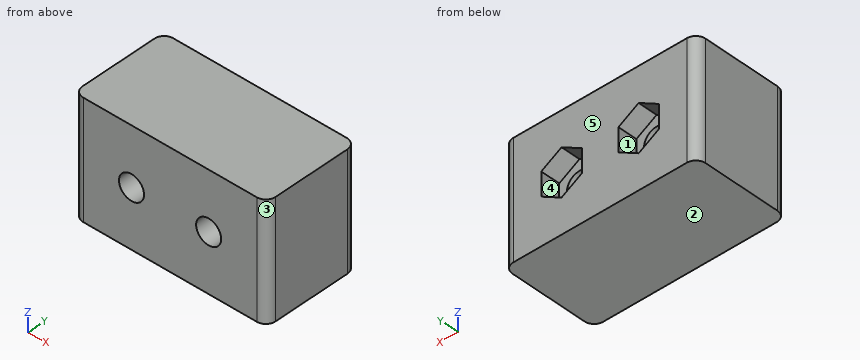
```python
from build123d import *

# Parameters (mm, degrees)
BOSS_EXTRUDE1_DEPTH = 6
SKETCH2_R           = 1.3
CUT_EXTRUDE1_DEPTH  = 10
CUT_EXTRUDE2_DEPTH  = 2


with BuildPart() as part:
    # Sketch1 → Boss-Extrude1 (new, symmetric)
    with BuildSketch(Plane.XY):
        with BuildLine():
            Line((-9, 0), (9, 0))
            ThreePointArc((9, 0), (9.707106781, 0.292893219), (10, 1))
            Line((10, 1), (10, 9))
            ThreePointArc((10, 9), (9.707106781, 9.707106781), (9, 10))
            Line((9, 10), (-9, 10))
            ThreePointArc((-9, 10), (-9.707106781, 9.707106781), (-10, 9))
            Line((-10, 9), (-10, 1))
            ThreePointArc((-10, 1), (-9.707106781, 0.292893219), (-9, 0))
        make_face()
    extrude(amount=BOSS_EXTRUDE1_DEPTH, both=True)

    # Sketch2 → Cut-Extrude1 (cut)
    with BuildSketch(Plane(origin=(0, 0, 0), x_dir=(1, 0, 0), z_dir=(0, 1, 0))):
        with Locations(Location((4, 0, 0), (0, 0, 270))):
            Circle(SKETCH2_R)
        with Locations(Location((-4, 0, 0), (0, 0, 270))):
            Circle(SKETCH2_R)
    extrude(amount=CUT_EXTRUDE1_DEPTH, mode=Mode.SUBTRACT)

    # Sketch3 → Cut-Extrude2 (cut)
    with BuildSketch(Plane(origin=(0, 10, 0), x_dir=(1, 0, 0), z_dir=(0, 1, 0))):
        Polygon((6.1, -1.212435565), (4, -2.424871131), (1.9, -1.212435565), (1.9, 1.212435565), (4, 2.424871131), (6.1, 1.212435565), align=None)
        Polygon((-1.9, -1.212435565), (-4, -2.424871131), (-6.1, -1.212435565), (-6.1, 1.212435565), (-4, 2.424871131), (-1.9, 1.212435565), align=None)
    extrude(amount=-CUT_EXTRUDE2_DEPTH, mode=Mode.SUBTRACT)


solid = part.part
```
CAD build for the part. Positions are in the model's coordinates, mm. Face numbers are marked on the shaded views. A direction names the side the tool comes from. Give positions to 0.01 mm unless a question says otherwise; leave off trailing zeros. Order: outer loops, then holes, each group sorted by start corner. A loop starts at its lowest first (then second) coordinate and runs counter-clockwise, first axis right, second up. Notation, with made-up numbers: M 37,-10.5 L 68,-10.5 A13 ccw 68,6.5 Z; hole C -9,61.5 d7. An arc over 180 degrees is marked long. Put each result on its own line as item: value. Start each with the question number.
(1) Mould opens along X. For the marked faces 1, 2 and 3 say: +X half, -X half, draft (parallel to the pull), parting line (faces both ways), or undercut.
(2) Which spindle directions (+Z, -Z, +X, -X, +Y, -Y) get a long thin tool onto all of the face, cutting with end or side? Do the marked faces 4 and 5. Say none if no direction does.
(3) Saw through at A-A, the plane z = 0. Write the cut outline in (x, y), then the cut area to 3 significant figures.
(4) Saw through at D-D, the plane y = 8.5. Write the cut outline in (x, z), then the cut area to 3 significant figures.
(5) Saw through at C-C, the plane x = 5.75. Write the cut outline in (y, z), then the cut area to 3 significant figures.
(6) Flat gauge pins, fed straight in: pin 1 Ø1.6 at (x, z) = (-4, 0) entering from -Y; pin 2 Ø0.6 at (y, z) = (9.5, 0.5) entering from +X. Where does each tip first touch, or does it go through?
(7) Saw through at B-B, the plane y = 6.25. Write the cut outline in (x, z), then the cut area to 3 significant figures.
(8) Drill centre lines: line 1 along X through (y, z) = (5.25, 0); line 2 along Z through (x, y) = (-4, 2.75); line 3 along X through (y, z) = (9.75, -0.5). Where is each one in solid material? Low to high.
Check result:
1. face 1: undercut
1. face 2: draft
1. face 3: +X half
2. face 4: +Y
2. face 5: +Z, -Z, +X, -X, +Y
3. outline: M -10,1 A1 ccw -9,0 L -5.3,0 L -5.3,8 L -6.1,8 L -6.1,10 L -9,10 A1 ccw -10,9 Z; M -2.7,0 L 2.7,0 L 2.7,8 L 1.9,8 L 1.9,10 L -1.9,10 L -1.9,8 L -2.7,8 Z; M 5.3,0 L 9,0 A1 ccw 10,1 L 10,9 A1 ccw 9,10 L 6.1,10 L 6.1,8 L 5.3,8 Z
3. area: 141 mm2
4. outline: M -10,-6 L 10,-6 L 10,6 L -10,6 Z; hole M -6.1,-1.21 L -4,-2.42 L -1.9,-1.21 L -1.9,1.21 L -4,2.42 L -6.1,1.21 Z; hole M 1.9,-1.21 L 4,-2.42 L 6.1,-1.21 L 6.1,1.21 L 4,2.42 L 1.9,1.21 Z
4. area: 209 mm2
5. outline: M 0,-6 L 10,-6 L 10,-1.41 L 8,-1.41 L 8,1.41 L 10,1.41 L 10,6 L 0,6 Z
5. area: 114 mm2
6. pin 1: passes through
6. pin 2: stops at x = 9.98
7. outline: M -10,-6 L 10,-6 L 10,6 L -10,6 Z; hole C -4,0 d2.6; hole C 4,0 d2.6
7. area: 229 mm2
8. line 1: x = -10 to -5.3, -2.7 to 2.7, 5.3 to 10
8. line 2: z = -6 to -1.3, 1.3 to 6
8. line 3: x = -9.66 to -6.1, -1.9 to 1.9, 6.1 to 9.66
